The listing builds one solid part. Answer for the finished solid, in the listing's coordinates (mm). Face numbers are marked on the shaded views. A direction names the side the tool comes from. Give positions to 0.01 mm unless a question says otherwise; leave off trailing zeros. Loops run counter-clockwise (first coordinate to the right, second up) from the corner with the lowest first, then second, coordinate; pieces in that order, holes last. Notation, with made-up numbers: M -2.5,-27 L 24.5,-27 A30 cw 24.5,-1 Z; hole C 1.5,52.5 d10. An arc over 180 degrees is marked long. One line per item, written item: value. Start each with the question number.
Q1. A cutting plane is placed at C-C, the plane y = -3. Determine the outline of the cut face in (x, z).
Q2. Flat-ended cylindrical pins translate along their axes: pin 1 (0.6 mm diameter, centred on y = -8, z = 11.5, fed in from -X); pin 2 (1.6 mm diameter, centred on x = -11, z = 0.5, fed in from -Y); pin 3 (4 mm diameter, centred on x = 14, z = 8, fed in from -Y). Find the tip coordinate at first contact, or state that the pin passes through.
Q3. A cutting plane is placed at A-A, the plane x = 15. Determine the outline of the cut face in (y, z), and give its area (3 significant figures).
Q4. Consider L1, parallel to X at y = 21.4, z = 6.25 (3 decimals); L2, parallel to Z at x = -15, y = 10; L3, parallel to Y at x = 7, z = 1.75. Determine where each line is inside the solid, lowest interval first.
Q5. A cutting plane is placed at B-B, the plane x = 1.25. Determine the outline of the cut face in (y, z), and give its area (3 significant figures).
Q6. For the marked faces 1, 2, 3 and 4, determine the directions among +Z, -Z, +X, -X, +Y, -Y from which every point of the face is accessible in a straight line to the end or side of a thin tool.
Q7. A cutting plane is placed at D-D, the plane x = -5.75. Determine the outline of the cut face in (y, z) (3 decimals).
Q8. The mould has two halves that part along Z. Classify the marked faces 5, 6 and 7: +Z half, -Z half, draft (parallel to the pull), parting line (faces both ways), or undercut.
from build123d import *

# Parameters (mm, degrees)
BOSS_EXTRUDE1_DEPTH = 12.5
BOSS_EXTRUDE2_DEPTH = 4.5
CHAMFER1_SIZE       = 2
SKETCH3_W           = 2
SKETCH3_H           = 2
SKETCH3_H_2         = 3.8
CUT_EXTRUDE1_DEPTH  = 2
CUT_EXTRUDE2_DEPTH  = 5
SKETCH5_R           = 2.5
BOSS_EXTRUDE3_DEPTH = 2.3
SKETCH6_R           = 0.625
CUT_EXTRUDE3_DEPTH  = 2.3


with BuildPart() as part:
    # Sketch1 → Boss-Extrude1 (new body)
    with BuildSketch(Plane.XY):
        Polygon((11.5, 9), (11.5, -9), (-11.5, -9), (-11.5, 9), (-16.5, 9), (-16.5, 11.5), (-11.5, 11.5), (-11.5, 15.5), (11.5, 15.5), (11.5, 11.5), (16.5, 11.5), (16.5, 9), align=None)
    extrude(amount=BOSS_EXTRUDE1_DEPTH)

    # Sketch2 → Boss-Extrude2 (add)
    with BuildSketch(Plane(origin=(0, 15.5, 0), x_dir=(1, 0, 0), z_dir=(0, 1, 0))):
        with BuildLine():
            ThreePointArc((-0.428571429, -4.071721331), (-11.5, -6.25), (-0.428571429, -8.428278669))
            ThreePointArc((-0.428571429, -8.428278669), (4, -6.25), (-0.428571429, -4.071721331))
        make_face()
    extrude(amount=BOSS_EXTRUDE2_DEPTH)

    # Chamfer1
    chamfer1_edges = [part.edges().sort_by_distance(p)[0] for p in [
        (-11.5, -9, 6.25),
    ]]
    chamfer(chamfer1_edges, length=CHAMFER1_SIZE)

    # Sketch3 → Cut-Extrude1 (cut)
    with BuildSketch(Plane.XZ.offset(9)):
        with Locations((-10.5, 1)):
            Rectangle(SKETCH3_W, SKETCH3_H)
        with Locations((-10.5, 11.5)):
            Rectangle(SKETCH3_W, SKETCH3_H)
        with Locations((-10.5, 6.25)):
            Rectangle(SKETCH3_W, SKETCH3_H_2)
    extrude(amount=-CUT_EXTRUDE1_DEPTH, mode=Mode.SUBTRACT)

    # Sketch4 → Cut-Extrude2 (cut)
    with BuildSketch(Plane(origin=(0, 11.5, 0), x_dir=(1, 0, 0), z_dir=(0, 1, 0))):
        with BuildLine():
            Line((16.145643924, -6.75), (17.156032055, -6.75))
            Line((17.156032055, -6.75), (17.156032055, -5.75))
            Line((17.156032055, -5.75), (16.145643924, -5.75))
            ThreePointArc((16.145643924, -5.75), (13.75, -6.25), (16.145643924, -6.75))
        make_face()
    cut_extrude2 = extrude(amount=-CUT_EXTRUDE2_DEPTH, mode=Mode.SUBTRACT)

    # Mirror1: Cut-Extrude2 across plane
    add(cut_extrude2.mirror(Plane.ZY), mode=Mode.SUBTRACT)

    # Sketch5 → Boss-Extrude3 (add)
    with BuildSketch(Plane(origin=(0, 20, 0), x_dir=(1, 0, 0), z_dir=(0, 1, 0))):
        with Locations((-5.75, -6.25)):
            Circle(SKETCH5_R)
    extrude(amount=BOSS_EXTRUDE3_DEPTH)

    # Sketch6 → Cut-Extrude3 (cut)
    with BuildSketch(Plane(origin=(0, 22.3, 0), x_dir=(1, 0, 0), z_dir=(0, 1, 0))):
        with Locations((-5.75, -6.25)):
            Circle(SKETCH6_R)
    extrude(amount=-CUT_EXTRUDE3_DEPTH, mode=Mode.SUBTRACT)


solid = part.part
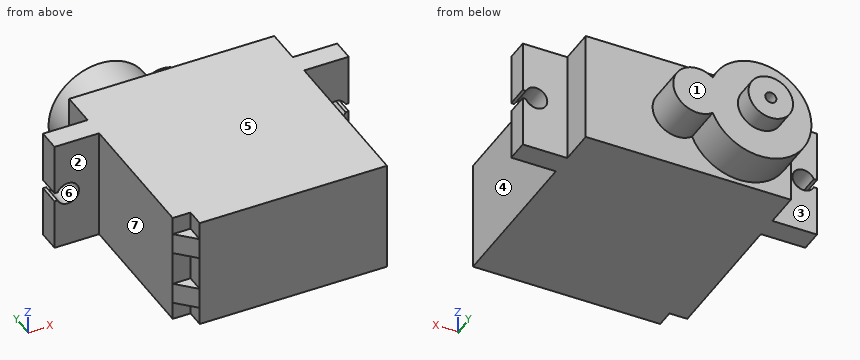
Answer block:
1. outline: M -11.5,0 L 11.5,0 L 11.5,12.5 L -11.5,12.5 Z
2. pin 1: x = -9.5
2. pin 2: y = -7
2. pin 3: y = 9
3. outline: M 9,0 L 11.5,0 L 11.5,5 L 9,5 Z; M 9,7.5 L 11.5,7.5 L 11.5,12.5 L 9,12.5 Z
3. area: 25.0 mm^2
4. L1: -8.25 to -6.375, -5.125 to -3.25
4. L2: 0 to 5, 7.5 to 12.5
4. L3: -9 to 15.5
5. outline: M -9,0 L 15.5,0 L 15.5,3.5 L 20,3.5 L 20,9 L 15.5,9 L 15.5,12.5 L -9,12.5 Z
5. area: 331 mm^2
6. face 1: +Y
6. face 2: +Z, -Z, -X, -Y
6. face 3: +Z, -Z, -X, +Y
6. face 4: +Z, -Z, +X, -Y
7. outline: M -9,0 L 15.5,0 L 15.5,0.5 L 20,0.5 L 20,3.75 L 22.3,3.75 L 22.3,5.625 L 20,5.625 L 20,6.875 L 22.3,6.875 L 22.3,8.75 L 20,8.75 L 20,12 L 15.5,12 L 15.5,12.5 L -9,12.5 Z
8. face 5: +Z half
8. face 6: undercut
8. face 7: draft
